Source: CAD feature listing. Evaluate the final solid. Frame: model axes, mm. Face numbers are marked on the shaded views. A direction names the side the tool comes from. Give positions to 0.01 mm unless a question says otherwise; leave off trailing zeros. Write each loop counter-clockwise with the first axis right and the second up, starting at its lowest first coordinate (ties: lowest second). Pieces come first, ordered by that corner, then holes.
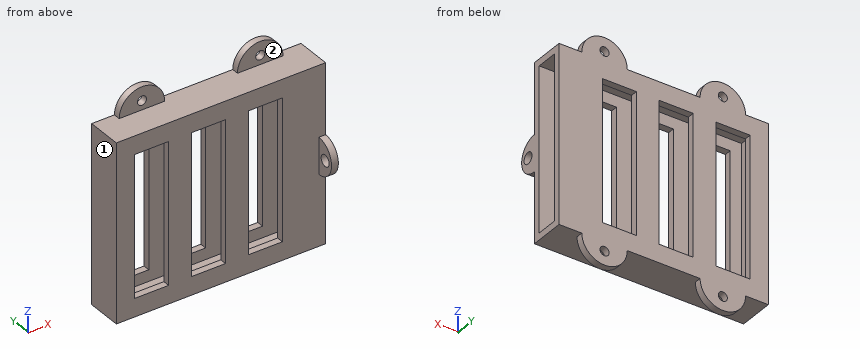
```python
from build123d import *

# Parameters (mm, degrees)
F0_W      = 92
F0_H      = 78
F1_DEPTH  = 15.5
F2_T      = -3
F4_DEPTH  = 3
F5_R      = 2
F6_DEPTH  = 25
F7_W      = 15
F7_H      = 62
F8_DEPTH  = 25
F10_DEPTH = 3
F11_R     = 2.5
F12_DEPTH = 5


# Not quite as in the source:
# - a feature names something its author has since deleted; it is built from what else it names


with BuildPart() as f1:
    # F0 (on Front) → F1 (new body)
    with BuildSketch(Plane.XZ):
        with Locations((-46, 39)):
            Rectangle(F0_W, F0_H)
    extrude(amount=F1_DEPTH)

    # F2
    f2_openings = [f1.faces().sort_by_distance(p)[0] for p in [
        (0, -7.75, 39),
    ]]
    offset(amount=F2_T, openings=f2_openings)

    # F3 (on face) → F4 (join)
    with BuildSketch(Plane(origin=(0, 0, 0), x_dir=(-1, 0, 0), z_dir=(0, 1, 0))):
        with BuildLine():
            Line((62, 78), (82, 78))
            ThreePointArc((82, 78), (72, 88), (62, 78))
        make_face()
        with BuildLine():
            ThreePointArc((62, 0), (72, -10), (82, 0))
            Line((82, 0), (62, 0))
        make_face()
        with BuildLine():
            Line((10, 78), (30, 78))
            ThreePointArc((30, 78), (20, 88), (10, 78))
        make_face()
        with BuildLine():
            ThreePointArc((10, 0), (20, -10), (30, 0))
            Line((30, 0), (10, 0))
        make_face()
    extrude(amount=-F4_DEPTH)

    # F5 (on face) → F6 (cut)
    with BuildSketch(Plane.XZ.offset(3)):
        with Locations((-72, 82)):
            Circle(F5_R)
        with Locations((-72, -4)):
            Circle(F5_R)
        with Locations((-20, 82)):
            Circle(F5_R)
        with Locations((-20, -4)):
            Circle(F5_R)
    extrude(amount=-F6_DEPTH, mode=Mode.SUBTRACT)

    # F7 (on face) → F8 (cut)
    with BuildSketch(Plane.XZ.offset(15.5)):
        with Locations((-76.5, 39)):
            Rectangle(F7_W, F7_H)
        with Locations((-51.5, 39)):
            Rectangle(F7_W, F7_H)
        with Locations((-26.5, 39)):
            Rectangle(F7_W, F7_H)
    extrude(amount=-F8_DEPTH, mode=Mode.SUBTRACT)

    # F9 (on face) → F10 (join)
    with BuildSketch(Plane.YZ):
        with BuildLine():
            Line((-15.5, 31), (-15.5, 47))
            ThreePointArc((-15.5, 47), (-23.5, 39), (-15.5, 31))
        make_face()
    extrude(amount=-F10_DEPTH)

    # F11 (on face) → F12 (cut)
    with BuildSketch(Plane.YZ):
        with Locations((-19.5, 39)):
            Circle(F11_R)
    extrude(amount=-F12_DEPTH, mode=Mode.SUBTRACT)


solid = f1.part
```
1. Cut plane A-A, the plane x = -49. Return the cut outline in (y, z), then the cut area to 3 significant figures.
2. Cut plane C-C, the plane y = -6.75. Return the cut outline in (x, z).
3. Access query for the marked faces 1 and 2. Directions: +Z, -Z, +X, -X, +Y, -Y. A direction counts if a zero-diameter tool reaches every point of the face in a straight line with its end or side. Return the directions, or none.
4. Cut plane D-D, the plane z = 25. State how many separate pieces and enclosed holes the cut face has, then the cut area to 4 significant figures.
5. Contact query for flat-ended pins moving along their axis: P1, Ø10, axis at x = -74, y = -10, coming from the +Z side; P2, Ø8, axis at x = -46.5, z = 43.5, coming from the -Y side; P3, Ø1.5, axis at x = -26.5, y = -13.5, coming from the -Z side. Output: stop coordinate, or through.
6. Cut plane B-B, the plane x = -66. Return the cut outline in (y, z).
7. Line query: L1, parallel to Z at x = -20, y = -2.2; L2, parallel to X at y = -14.75, z = 40.5; L3, parallel to Z at x = -25, y = -14.5. Output: solid intervals per line, ascending.
Response values:
1. outline: (-15.5, 0) - (0, 0) - (0, 8) - (-3, 8) - (-3, 3) - (-12.5, 3) - (-12.5, 8) - (-15.5, 8) - close; (-15.5, 70) - (-12.5, 70) - (-12.5, 75) - (-3, 75) - (-3, 70) - (0, 70) - (0, 78) - (-15.5, 78) - close
1. area: 153 mm2
2. outline: (-92, 0) - (0, 0) - (0, 3) - (-89, 3) - (-89, 75) - (0, 75) - (0, 78) - (-92, 78) - close
3. face 1: +Z, -Z, -X, +Y, -Y
3. face 2: +Z, +X, -X, -Y
4. separate pieces: 7
4. enclosed holes: 0
4. area: 310.5 mm2
5. P1: stops at z = 78
5. P2: stops at y = -15.5
5. P3: stops at z = 0
6. outline: (-15.5, 0) - (-3, 0) - (-3, -8) - (0, -8) - (0, 86) - (-3, 86) - (-3, 78) - (-15.5, 78) - close; hole (-12.5, 3) - (-3, 3) - (-3, 75) - (-12.5, 75) - close
7. L1: z = -10 to -6, -2 to 8, 70 to 80, 84 to 88
7. L2: x = -92 to -84, -69 to -59, -44 to -34, -19 to 0
7. L3: z = 0 to 8, 70 to 78
